Autodesk Inventor part; units mm, degrees
ref_plane "YZ Plane" through (0, 0, 0) normal (1, 0, 0) x (0, 1, 0)
ref_plane "XZ Plane" through (0, 0, 0) normal (0, 1, 0) x (-1, 0, 0)
ref_plane "XY Plane" through (0, 0, 0) normal (0, 0, 1) x (1, 0, 0)
sketch "Skizze1" plane through (0, 0, 0) normal (0, 0, 1) x (1, 0, 0)
  circle A0 centre (0, 0) radius 11.5
  circle A1 centre (0, 0) radius 8.5 construction
  circle A2 centre (0, 8.5) radius 1.15
  circle A3 centre (0, -8.5) radius 1.15
  line L0 (0, 16.1) -> (0, -16.1) construction
  circle A4 centre (0, 0) radius 6
  dimension "MEncoder_OuterDia" = 23
  dimension "MEncoder_FixationHole_Dia" = 17
  dimension "d2" = 2.3
  dimension "d3" = 2.3
  dimension "MagneticEnc_Magnet_PassHole" = 12
extrude "Montageplatte" add sketch "Skizze1" along normal blind 2
sketch "Skizze2" plane through (0, 0, 2) normal (0, 0, 1) x (1, 0, 0)
  line L0 (-10.4523, 1) -> (-11.4564, 1)
  line L1 (-11.4564, -1) -> (-10.4523, -1)
  line L2 (-10.4523, 1) -> (-11.5781, -1) construction
  line L3 (-11.5781, 1) -> (-10.4523, -1) construction
  line L4 (-16.1937, 0) -> (16.1156, 0) construction
  circle A0 centre (0, 0) radius 11.5 construction
  circle A1 centre (0, 0) radius 11.5 construction
  arc A2 (-11.4564, 1) -> (-11.4564, -1) centre (0, 0) ccw
  circle A3 centre (0, 0) radius 10.5 construction
  arc A4 (-10.4523, 1) -> (-10.4523, -1) centre (0, 0) ccw
  line L5 (4.3601, -9.5519) -> (4.8622, -10.4216)
  line L6 (6.5942, -9.4216) -> (6.0922, -8.5519)
  line L7 (4.3601, -9.5519) -> (6.6551, -9.5269) construction
  line L8 (4.923, -10.5269) -> (6.0922, -8.5519) construction
  arc A5 (4.8622, -10.4216) -> (6.5942, -9.4216) centre (0, 0) ccw
  arc A6 (4.3601, -9.5519) -> (6.0922, -8.5519) centre (0, 0) ccw
  line L9 (6.0922, 8.5519) -> (6.5942, 9.4216)
  line L10 (4.8622, 10.4216) -> (4.3601, 9.5519)
  line L11 (6.0922, 8.5519) -> (4.923, 10.5269) construction
  line L12 (6.6551, 9.5269) -> (4.3601, 9.5519) construction
  arc A7 (6.5942, 9.4216) -> (4.8622, 10.4216) centre (0, 0) ccw
  arc A8 (6.0922, 8.5519) -> (4.3601, 9.5519) centre (0, 0) ccw
  point P0 (-11.0152, 0)
  point P1 (-11.0152, 0)
  point P2 (-11.0152, 0)
  point P3 (-11.5, 0)
  point P4 (5.5076, -9.5394)
  point P5 (5.5076, -9.5394)
  point P6 (5.5076, -9.5394)
  point P7 (5.75, -9.9593)
  point P8 (5.5076, 9.5394)
  point P9 (5.5076, 9.5394)
  point P10 (5.5076, 9.5394)
  point P11 (5.75, 9.9593)
  dimension "d10" = 2
  dimension "d17" = 2
  dimension "d24" = 1
  dimension "d25" = 1
  dimension "d36" = 21
  dimension "d39" = 360
extrude "Schnaphebel" add sketch "Skizze2" along normal blind 8
sketch "Skizze3" plane through (0, 0, 2) normal (0, 0, 1) x (1, 0, 0)
  circle A0 centre (0, 0) radius 10.5
  line L0 (4.8622, -10.4216) -> (4.3601, -9.5519)
  arc A1 (4.3601, -9.5519) -> (6.0922, -8.5519) centre (0, 0) ccw
  line L1 (6.0922, -8.5519) -> (6.5942, -9.4216)
  arc A2 (6.5942, -9.4216) -> (6.5942, 9.4216) centre (0, 0) ccw
  line L2 (6.5942, 9.4216) -> (6.0922, 8.5519)
  arc A3 (6.0922, 8.5519) -> (4.3601, 9.5519) centre (0, 0) ccw
  line L3 (4.3601, 9.5519) -> (4.8622, 10.4216)
  arc A4 (4.8622, 10.4216) -> (-11.4564, 1) centre (0, 0) ccw
  line L4 (-11.4564, 1) -> (-10.4523, 1)
  arc A5 (-10.4523, 1) -> (-10.4523, -1) centre (0, 0) ccw
  line L5 (-10.4523, -1) -> (-11.4564, -1)
  arc A6 (-11.4564, -1) -> (4.8622, -10.4216) centre (0, 0) ccw
  circle A7 centre (0, 8.5) radius 1.15
  circle A8 centre (0, -8.5) radius 1.15
  circle A9 centre (0, 0) radius 6
  dimension "d41" = 21
extrude "Sensorabdeckung" add sketch "Skizze3" along normal blind 16 contours A0 L2 A2 L1 | A0 L4 A4 L3 | L0 A6 L5 A0
sketch "Skizze4" plane through (0, 0, 18) normal (0, 0, 1) x (1, 0, 0)
  circle A0 centre (0, 0) radius 10.5
  arc A1 (4.3601, 9.5519) -> (-10.4523, 1) centre (0, 0) ccw
extrude "Sensorabdeckung Deckel" add sketch "Skizze4" against normal blind 3
properties part number "Magnetic Encoder" material "Polylactid (PLA) black"
Input: part model. Units: mm. Frame: model coordinates. A direction names the side the tool comes from. Coordinates: 2 decimals unless noted, no trailing zeros. Write each loop counter-clockwise with the first axis right and the second up, starting at its lowest first coordinate (ties: lowest second). Pieces come first, ordered by that corner, then holes.
1) Section C-C on z = 10.75. Output: boundary loops of the cut face in (x, y), and give its area (3 significant figures).
2) Section D-D on x = -0.75. Output: boundary loops of the cut face in (y, z).
3) Section B-B on z = 8.5. Output: boundary loops of the cut face in (x, y), and give its area (3 significant figures).
4) Pin query (flat end, axial travel): pin 1 Ø4 at (y, z) = (8, 11) entering from +X; pin 2 Ø8 at (y, z) = (5, 7.5) entering from -X; pin 3 Ø1.5 at (x, y) = (6, 10) entering from +Z. Return the tip coordinate at first contact, or that it passes through.
5) Set-up query: faces 4 (the cylindrical face through (-5.13, -9.16, 8.41)), 5 (the flat face through (5.5, -9.5, 10)), 6 (the cylindrical face through (-6, 0, 1)). Return all of +Z, -Z, +X, -X, +Y, -Y with unobstructed straight access to the full face (end or side cutting, diameter ignored); none if empty.
6) Mould query, pull axis X, two halves, no side actions, for faces 1 (the cylindrical face through (5.262, 9.086, 16.521)), 2 (the cylindrical face through (5.762, -9.952, 5.944)), 3 (the flat face through (5, -5, 0)). Classes: pulls with the +X half, pulls with the -X half, needs draft (parallel to the pull), parting line crosses it, or undercut.
7) Section A-A on y = 0. Output: boundary loops of the cut face in (x, z), and give its area (3 significant figures).
8) Material intervals for line 1 along Y through (x, z) = (0, 0.5); line 2 along Z through (x, y) = (8.5, -5.25); line 3 along Y through (x, z) = (8.75, 2.75), sorted ascending.
Check result:
1. outline: (-11.46, -1) arc R11.5 ccw to (4.86, -10.42) - (4.36, -9.55) arc R10.5 cw to (-10.45, -1) - close; (-11.46, 1) - (-10.45, 1) arc R10.5 cw to (4.36, 9.55) - (4.86, 10.42) arc R11.5 ccw to start; (6.09, -8.55) - (6.59, -9.42) arc R11.5 ccw to (6.59, 9.42) - (6.09, 8.55) arc R10.5 cw to start
1. area: 63.1 mm2
2. outline: (-11.48, 0) - (-9.37, 0) - (-9.37, 2) - (-10.47, 2) - (-10.47, 15) - (10.47, 15) - (10.47, 2) - (9.37, 2) - (9.37, 0) - (11.48, 0) - (11.48, 18) - (-11.48, 18) - close; (-7.63, 0) - (-5.95, 0) - (-5.95, 2) - (-7.63, 2) - close; (5.95, 0) - (7.63, 0) - (7.63, 2) - (5.95, 2) - close
3. outline: (-11.46, -1) arc R11.5 ccw to (4.86, -10.42) arc R11.5 ccw to (6.59, -9.42) arc R11.5 ccw to (6.59, 9.42) arc R11.5 ccw to (4.86, 10.42) arc R11.5 ccw to (-11.46, 1) arc R11.5 ccw to start; hole (4.36, -9.55) arc R10.5 ccw to (6.09, -8.55) arc R10.5 ccw to (6.09, 8.55) arc R10.5 ccw to (4.36, 9.55) arc R10.5 ccw (long way) to start
3. area: 69.1 mm2
4. pin 1: stops at x = 9.81
4. pin 2: stops at x = -11.46
4. pin 3: stops at z = 10
5. face 4: none
5. face 5: +Z
5. face 6: -Z
6. face 1: undercut
6. face 2: pulls with the +X half
6. face 3: needs draft
7. outline: (-11.5, 0) - (-6, 0) - (-6, 2) - (-10.5, 2) - (-10.5, 10) - (-11.5, 10) - close; (-10.5, 15) - (10.5, 15) - (10.5, 2) - (6, 2) - (6, 0) - (11.5, 0) - (11.5, 18) - (-10.5, 18) - close
7. area: 109 mm2
8. line 1: y = -11.5 to -9.65, -7.35 to -6, 6 to 7.35, 9.65 to 11.5
8. line 2: z = 0 to 2, 15 to 18
8. line 3: y = -7.46 to -5.8, 5.8 to 7.46
